from build123d import *

# Parameters (mm, degrees)
SKETCH1_R      = 3.302
EXTRUDE1_DEPTH = 3.175


with BuildPart() as part:
    # Sketch1 → Extrude1 (new body)
    with BuildSketch(Plane.XY):
        Polygon((-12.7, 12.7), (-3.175, 12.7), (-3.175, 9.525), (3.175, 9.525), (3.175, 12.7), (12.7, 12.7), (12.7, 3.175), (9.525, 3.175), (9.525, -3.175), (12.7, -3.175), (12.7, -12.7), (3.175, -12.7), (3.175, -9.525), (-3.175, -9.525), (-3.175, -12.7), (-12.7, -12.7), (-12.7, -3.175), (-9.525, -3.175), (-9.525, 3.175), (-12.7, 3.175), align=None)
        Circle(SKETCH1_R, mode=Mode.SUBTRACT)
    extrude(amount=EXTRUDE1_DEPTH)


solid = part.part
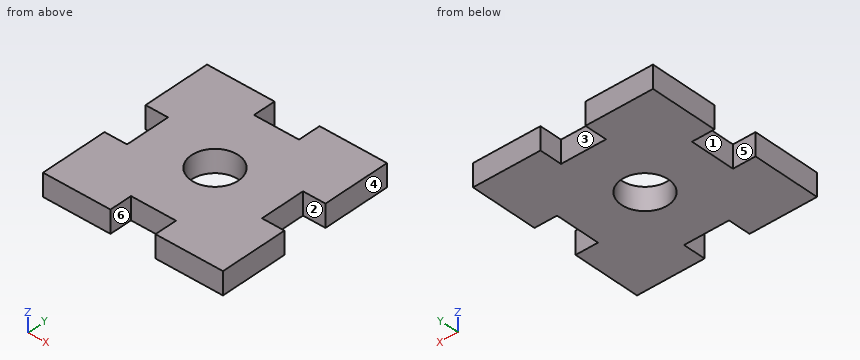
Part model, mm, in its own coordinate system. Face numbers are marked on the shaded views. A direction names the side the tool comes from. Give positions to 0.01 mm unless a question says otherwise; leave off trailing zeros. Write each loop counter-clockwise with the first axis right and the second up, starting at its lowest first coordinate (ties: lowest second). Pieces come first, ordered by that corner, then holes.
1) Which spindle directions (+Z, -Z, +X, -X, +Y, -Y) get a long thin tool onto all of the face, cutting with end or side? Do the marked faces 1, 2 and 3. Say none if no direction does.
Resolved:
face 1: +Z, -Z, -X
face 2: +Z, -Z, +X
face 3: +Z, -Z, +Y
2) Probe L1, parallel to Y at x = 0, z = 0.85 (3 decimals); L2, parallel to Y at x = 10.5, z = 0.4 (3 decimals). List the from-to ranges inside material, lowest first.
Resolved:
L1: y = -9.525 to -3.302, 3.302 to 9.525
L2: y = -12.7 to -3.175, 3.175 to 12.7
3) Pin check, flat tips, straight feed: pin 1 (1.6 mm diameter, centred on y = 1.5, z = 1.5, fed in from +X) (3 decimals); pin 2 (1 mm diameter, centred on y = -1.5, z = 1.5, fed in from -X) (3 decimals). Stop position of each tip, or through.
Resolved:
pin 1: stops at x = 9.525
pin 2: stops at x = -9.525
4) Two-plate mould, pull along X, no slides. Class the marked faces 4, 5 and 6: released by +X, released by -X, zero draft, split by the parting line, or undercut.
Resolved:
face 4: released by +X
face 5: zero draft
face 6: undercut
5) Cut at B-B on z = 0.5. Write the cut outline in (x, y) (3 decimals).
Resolved:
outline: (-12.7, -12.7) - (-3.175, -12.7) - (-3.175, -9.525) - (3.175, -9.525) - (3.175, -12.7) - (12.7, -12.7) - (12.7, -3.175) - (9.525, -3.175) - (9.525, 3.175) - (12.7, 3.175) - (12.7, 12.7) - (3.175, 12.7) - (3.175, 9.525) - (-3.175, 9.525) - (-3.175, 12.7) - (-12.7, 12.7) - (-12.7, 3.175) - (-9.525, 3.175) - (-9.525, -3.175) - (-12.7, -3.175) - close; hole circle Ø6.604 at (0, 0)
6) Cut at A-A on y = 0. Write the cut outline in (x, z) (3 decimals).
Resolved:
outline: (-9.525, 0) - (-3.302, 0) - (-3.302, 3.175) - (-9.525, 3.175) - close; (3.302, 0) - (9.525, 0) - (9.525, 3.175) - (3.302, 3.175) - close
